Read the model definition and answer for the solid it produces. Units are mm, in the model's axes. Face numbers are marked on the shaded views. A direction names the side the tool comes from. Coordinates: 2 decimals unless noted, no trailing zeros. Order: outer loops, then holes, each group sorted by start corner. A loop starts at its lowest first (then second) coordinate and runs counter-clockwise, first axis right, second up. Notation, with made-up numbers: (72.5, 11.25) - (76.5, 11.25) arc R18 cw to (76.5, 36.25) - close; hole circle Ø5 at (16.25, 15). An arc over 180 degrees is marked (long way). Write item = value, one per line.
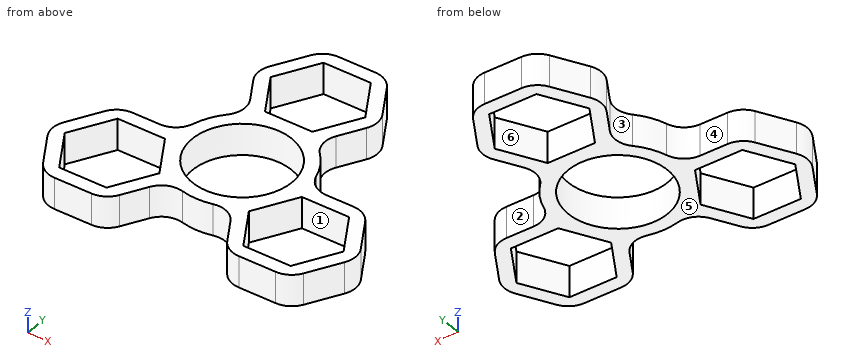
from build123d import *

# Parameters (mm, degrees)
F0_R     = 11.1
F1_DEPTH = 7


with BuildPart() as f1:
    # F0 (on Top) → F1 (new body)
    with BuildSketch(Plane.XY):
        with BuildLine():
            Line((4.058772, 35.45), (-4.058772, 35.45))
            ThreePointArc((-4.058772, 35.45), (-6.558772, 34.780127), (-8.388899, 32.95))
            Line((-8.388899, 32.95), (-12.447672, 25.92))
            ThreePointArc((-12.447672, 25.92), (-13.117545, 23.42), (-12.447672, 20.92))
            Line((-12.447672, 20.92), (-9.4492, 15.726494))
            ThreePointArc((-9.4492, 15.726494), (-8.815683, 12.624629), (-10.172173, 9.764061))
            ThreePointArc((-10.172173, 9.764061), (-12.210958, 7.05), (-13.542012, 3.92733))
            ThreePointArc((-13.542012, 3.92733), (-15.341091, 1.322291), (-18.344143, 0.32))
            Line((-18.344143, 0.32), (-24.341087, 0.32))
            ThreePointArc((-24.341087, 0.32), (-26.841087, -0.349873), (-28.671214, -2.18))
            Line((-28.671214, -2.18), (-32.729987, -9.21))
            ThreePointArc((-32.729987, -9.21), (-33.39986, -11.71), (-32.729987, -14.21))
            Line((-32.729987, -14.21), (-28.671214, -21.24))
            ThreePointArc((-28.671214, -21.24), (-26.841087, -23.070127), (-24.341087, -23.74))
            Line((-24.341087, -23.74), (-16.223543, -23.74))
            ThreePointArc((-16.223543, -23.74), (-13.723543, -23.070127), (-11.893416, -21.24))
            Line((-11.893416, -21.24), (-8.894944, -16.046494))
            ThreePointArc((-8.894944, -16.046494), (-6.525408, -13.94692), (-3.369838, -13.691391))
            ThreePointArc((-3.369838, -13.691391), (0, -14.1), (3.369838, -13.691391))
            ThreePointArc((3.369838, -13.691391), (6.525408, -13.94692), (8.894944, -16.046494))
            Line((8.894944, -16.046494), (11.893416, -21.24))
            ThreePointArc((11.893416, -21.24), (13.723543, -23.070127), (16.223543, -23.74))
            Line((16.223543, -23.74), (24.341087, -23.74))
            ThreePointArc((24.341087, -23.74), (26.841087, -23.070127), (28.671214, -21.24))
            Line((28.671214, -21.24), (32.729987, -14.21))
            ThreePointArc((32.729987, -14.21), (33.39986, -11.71), (32.729987, -9.21))
            Line((32.729987, -9.21), (28.671214, -2.18))
            ThreePointArc((28.671214, -2.18), (26.841087, -0.349873), (24.341087, 0.32))
            Line((24.341087, 0.32), (18.344143, 0.32))
            ThreePointArc((18.344143, 0.32), (15.341091, 1.322291), (13.542012, 3.92733))
            ThreePointArc((13.542012, 3.92733), (12.210958, 7.05), (10.172173, 9.764061))
            ThreePointArc((10.172173, 9.764061), (8.815683, 12.624629), (9.4492, 15.726494))
            Line((9.4492, 15.726494), (12.447672, 20.92))
            ThreePointArc((12.447672, 20.92), (13.117545, 23.42), (12.447672, 25.92))
            Line((12.447672, 25.92), (8.388899, 32.95))
            ThreePointArc((8.388899, 32.95), (6.558772, 34.780127), (4.058772, 35.45))
        make_face()
        Polygon((-30.709261, -11.71), (-25.495788, -2.68), (-15.068842, -2.68), (-9.855369, -11.71), (-15.068842, -20.74), (-25.495788, -20.74), align=None, mode=Mode.SUBTRACT)
        Polygon((25.495788, -20.74), (15.068842, -20.74), (9.855369, -11.71), (15.068842, -2.68), (25.495788, -2.68), (30.709261, -11.71), align=None, mode=Mode.SUBTRACT)
        Circle(F0_R, mode=Mode.SUBTRACT)
        Polygon((-10.426946, 23.42), (-5.213473, 32.45), (5.213473, 32.45), (10.426946, 23.42), (5.213473, 14.39), (-5.213473, 14.39), align=None, mode=Mode.SUBTRACT)
    extrude(amount=F1_DEPTH)


solid = f1.part
1) Determine the mould class of the marked faces 4, 5 and 6 for opening direction Y: pulls with the +Y half, pulls with the -Y half, needs draft (parallel to the pull), parting line crosses it, or undercut.
Returned:
face_4 = pulls with the +Y half
face_5 = needs draft
face_6 = undercut
2) For the marked faces 1, 2 and 3, determine the directions among +Z, -Z, +X, -X, +Y, -Y from which every point of the face is accessible in a straight line to the end or side of a thin tool.
Returned:
face_1 = +Z, -Z
face_2 = +Z, -Z, +X, +Y
face_3 = +Z, -Z, -X
3) Flat-ended cylindrical pins translate along their axes: pin 1 Ø2 at (x, z) = (-22.5, 3.5) entering from +Y; pin 2 Ø8 at (x, y) = (-18.5, -7.5) entering from -Z. Find the tip coordinate at first contact, or state that the pin passes through.
Returned:
pin_1 = 0.32
pin_2 = through
4) The part is cut by section B-B (y = -7.5). Determine the outline of the cut face in (x, z), and give its area (3 significant figures).
Returned:
outline = (-31.74, 0) - (-28.28, 0) - (-28.28, 7) - (-31.74, 7) - close; (-12.29, 0) - (-8.18, 0) - (-8.18, 7) - (-12.29, 7) - close; (8.18, 0) - (12.29, 0) - (12.29, 7) - (8.18, 7) - close; (28.28, 0) - (31.74, 0) - (31.74, 7) - (28.28, 7) - close
area = 106 mm^2
5) The part is cut by section C-C (z = 6). Count the separate pieces of the cut face and the enclosed holes in it, and give its area (3 significant figures).
Returned:
separate_pieces = 1
enclosed_holes = 4
area = 808 mm^2
6) The part is cut by section A-A (x = 0). Determine the outline of the cut face in (y, z).
Returned:
outline = (-14.1, 0) - (-11.1, 0) - (-11.1, 7) - (-14.1, 7) - close; (11.1, 0) - (14.39, 0) - (14.39, 7) - (11.1, 7) - close; (32.45, 0) - (35.45, 0) - (35.45, 7) - (32.45, 7) - close
7) The part is cut by section D-D (y = 13). Determine the outline of the cut face in (x, z).
Returned:
outline = (-8.78, 0) - (8.78, 0) - (8.78, 7) - (-8.78, 7) - close
8) Straight lines are drawn through the part: line 1 along Y through (x, z) = (0, 4.5); line 2 along Y through (x, z) = (23, 5.75); line 3 along X through (y, z) = (-12, 4). For each, find the intervals that lie inside material, in ascending order. Write a range as from..to.
Returned:
line_1 = -14.1..-11.1, 11.1..14.39, 32.45..35.45
line_2 = -23.74..-20.74, -2.68..0.32
line_3 = -33.39..-30.54, -10.02..10.02, 30.54..33.39
